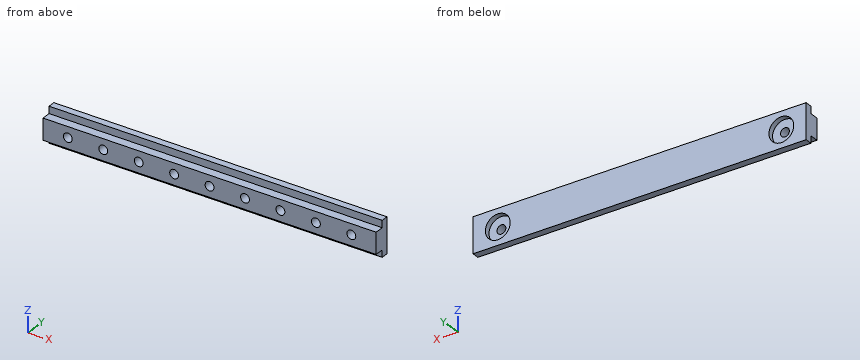
from build123d import *

# Parameters (mm, degrees)
SKETCH1_W          = 94
SKETCH1_H          = 4.5
MAIN_DEPTH         = 5
SKETCH4_W          = 94
SKETCH4_H          = 2.5
WINDOWSLOT1_DEPTH  = 2
SKETCH6_R          = 1.25
CUT_EXTRUDE2_DEPTH = 3
LPATTERN1_COUNT    = 9
LPATTERN1_PITCH    = 10
SKETCH7_R          = 3.5
CUT_EXTRUDE4_DEPTH = 1.5


with BuildPart() as part:
    # Sketch1 → Main (new body, symmetric)
    with BuildSketch(Plane.XY):
        with Locations((0, -2.25)):
            Rectangle(SKETCH1_W, SKETCH1_H)
    extrude(amount=MAIN_DEPTH, both=True)

    # Sketch4 → WindowSlot1 (cut)
    with BuildSketch(Plane.XY.offset(5)):
        with Locations((0, -3.25)):
            Rectangle(SKETCH4_W, SKETCH4_H)
    windowslot1 = extrude(amount=-WINDOWSLOT1_DEPTH, mode=Mode.SUBTRACT)

    # Mirror1: WindowSlot1 across plane
    add(windowslot1.mirror(Plane.XY), mode=Mode.SUBTRACT)

    # Sketch6 → Cut-Extrude2 (cut)
    with BuildSketch(Plane.ZX.offset(-4.5)):
        with Locations((0, 40)):
            Circle(SKETCH6_R)
    cut_extrude2 = extrude(amount=CUT_EXTRUDE2_DEPTH, mode=Mode.SUBTRACT)

    # LPattern1: Cut-Extrude2 ×9
    with Locations(*[(-i * LPATTERN1_PITCH, 0, 0) for i in range(1, LPATTERN1_COUNT)]):
        add(cut_extrude2, mode=Mode.SUBTRACT)

    # Sketch7 → Cut-Extrude4 (cut)
    with BuildSketch(Plane.ZX):
        with Locations((0, 40)):
            Circle(SKETCH7_R)
        with Locations((0, -40)):
            Circle(SKETCH7_R)
    extrude(amount=-CUT_EXTRUDE4_DEPTH, mode=Mode.SUBTRACT)


solid = part.part
Work out the finished part from the listing and answer in its coordinate system (mm). Coordinates: 2 decimals unless noted, no trailing zeros. Order: outer loops, then holes, each group sorted by start corner. A loop starts at its lowest first (then second) coordinate and runs counter-clockwise, first axis right, second up. Notation, with made-up numbers: (28, 12) - (34, 12) arc R13 ccw to (34, 27) - close; hole circle Ø3 at (86.5, -2.5). An arc over 180 degrees is marked (long way). Put each result on its own line as item: value. Start each with the question number.
1) Find section B-B (y = -2.7). State how many separate pieces and enclosed holes the cut face has, plus the area to 3 significant figures.
2) Find section C-C (x = -30). Give the vertices of the cut face in (y, z).
3) Find section A-A (x = 40). Give the vertices of the cut face in (y, z).
4) Find the intervals of material crossed by line 1 (X direction, y = -0.3, z = 0.25); line 2 (X direction, y = -0.5, z = 1.25); line 3 (Z direction, x = -26.5, y = -3.1), in increasing order. Write a range as from..to.
5) Flat-ended cylindrical pins translate along their axes: pin 1 (2 mm diameter, centred on x = 0, z = 0, fed in from -Y); pin 2 (2 mm diameter, centred on x = -40, z = 0, fed in from +Y); pin 3 (1.6 mm diameter, centred on x = -21, z = -4, fed in from -Y). Find the tip coordinate at first contact, or state that the pin passes through.
Results list:
1. separate pieces: 1
1. enclosed holes: 9
1. area: 520 mm^2
2. outline: (-4.5, -3) - (-2, -3) - (-2, -5) - (0, -5) - (0, 5) - (-2, 5) - (-2, 3) - (-4.5, 3) - (-4.5, 1.25) - (-1.5, 1.25) - (-1.5, -1.25) - (-4.5, -1.25) - close
3. outline: (-4.5, -3) - (-2, -3) - (-2, -5) - (0, -5) - (0, -3.5) - (-1.5, -3.5) - (-1.5, -1.25) - (-4.5, -1.25) - close; (-4.5, 1.25) - (-1.5, 1.25) - (-1.5, 3.5) - (0, 3.5) - (0, 5) - (-2, 5) - (-2, 3) - (-4.5, 3) - close
4. line 1: x = -47..-43.49, -36.51..36.51, 43.49..47
4. line 2: x = -47..-43.27, -36.73..36.73, 43.27..47
4. line 3: z = -3..3
5. pin 1: stops at y = -1.5
5. pin 2: passes through
5. pin 3: stops at y = -2
